Autodesk Inventor part; units mm, degrees
ref_plane "YZ Plane" through (0, 0, 0) normal (1, 0, 0) x (0, 1, 0)
ref_plane "XZ Plane" through (0, 0, 0) normal (0, 1, 0) x (-1, 0, 0)
ref_plane "XY Plane" through (0, 0, 0) normal (0, 0, 1) x (1, 0, 0)
sketch "Sketch1" plane through (0, 0, 0) normal (0, 1, 0) x (-1, 0, 0)
  line L0 (25, 25) -> (-25, 25)
  line L1 (-25, 25) -> (-25, -25)
  line L2 (-25, -25) -> (25, -25)
  line L3 (25, -25) -> (25, 25)
  line L4 (25, 25) -> (-25, -25) construction
  line L5 (-25, 25) -> (25, -25) construction
  point P0 (0, 0)
  dimension "d0" = 50
  dimension "d1" = 50
extrude "Extrusion1" add sketch "Sketch1" along normal mid plane 50
chamfer "Chamfer1" distance 5 angle 45 12 edges at (25, 0, -25) (0, 25, -25) (-25, 0, -25) (-25, 25, 0) (-25, 0, 25) (25, 0, 25) (0, -25, -25) (-25, -25, 0) (0, -25, 25) (25, -25, 0) (25, 25, 0) (0, 25, 25)
properties part number "ElementaryCube" material "Silver"
Part model, mm, in its own coordinate system. Give positions to 0.01 mm unless a question says otherwise; leave off trailing zeros. Loops run counter-clockwise (first coordinate to the right, second up) from the corner with the lowest first, then second, coordinate; pieces in that order, holes last. Notation, with made-up numbers: M 37.25,84.25 L 53.25,84.25 A13 cw 53.25,97.25 Z; hole C 3.5,60.5 d11. An arc over 180 degrees is marked long. Put each result on its own line as item: value. Start each with the question number.
1) Probe probe 1 along Z at (x, y) = (-9.5, 22); probe 2 along X at (y, z) = (23.5, 5). List the from-to ranges inside material, lowest first.
2) Saw through at A-A (x = 21.5). List the corners of the cut face in (y, z), then the cut area to 3 significant figures.
3) Saw through at B-B (y = 17). List the corners of the cut face in (x, z), then the cut area to 3 significant figures.
Numbers:
1. probe 1: -23 to 23
1. probe 2: -21.5 to 21.5
2. outline: M -23.5,-20 L -20,-23.5 L 20,-23.5 L 23.5,-20 L 23.5,20 L 20,23.5 L -20,23.5 L -23.5,20 Z
2. area: 2,180 mm^2
3. outline: M -25,-20 L -20,-25 L 20,-25 L 25,-20 L 25,20 L 20,25 L -20,25 L -25,20 Z
3. area: 2,450 mm^2
